Can you work these out from the model? Positions are in its coordinate system, mm. Give positions to 0.01 mm unless a question says otherwise; leave off trailing zeros. Write each loop counter-clockwise with the first axis right and the second up, starting at its lowest first coordinate (ties: lowest second). Pieces come first, ordered by that corner, then holes. Notation, with made-up numbers: (71, 45) - (122, 45) arc R6 ccw to (122, 54) - close; hole circle Ø1 at (-1, -32). An arc over 180 degrees is marked (long way). Use a Markdown table: item, result. Add a question column.
```python
from build123d import *

# Parameters (mm, degrees)
F0_R     = 25.1418135505
F1_DEPTH = 32.512
F2_T     = -2.54


# Not quite as in the source:
# - a fillet or chamfer that OpenCascade refuses, or shapes differently, is made with other operations: its cross-section is extruded or revolved along the edge and cut away or added


with BuildPart() as f1:
    # F0 (on Top) → F1 (new body)
    with BuildSketch(Plane.XY):
        Circle(F0_R)
    extrude(amount=F1_DEPTH)

    # F2
    f2_openings = [f1.faces().sort_by_distance(p)[0] for p in [
        (0, 0, 32.512),
    ]]
    offset(amount=F2_T, openings=f2_openings)

    # F3: fillet of radius 5.08 on 3 edges, made by hand

    # F3_s1 → F3_t2 (revolve, cut)
    with BuildSketch(Plane.XZ):
        with BuildLine():
            ThreePointArc((25.1418135505, 28.1125909488), (24.4612226018, 30.6525909488), (22.6018135505, 32.512))
            Line((22.6018135505, 32.512), (22.6526135505, 32.599988181))
            ThreePointArc((22.6526135505, 32.599988181), (23.8718135505, 32.6136), (25.1418135505, 32.6136))
            Line((25.1418135505, 32.6136), (25.2434135505, 32.512))
            Line((25.2434135505, 32.512), (25.2434135505, 28.1125909488))
            Line((25.2434135505, 28.1125909488), (25.1418135505, 28.1125909488))
        make_face()
    revolve(axis=Axis((0, 0, 32.512), (0, 0, 1)), mode=Mode.SUBTRACT)

    # F3_s3 → F3_t4 (revolve, cut)
    with BuildSketch(Plane.XZ):
        with BuildLine():
            ThreePointArc((25.1418135505, 5.08), (23.653915999, 1.4878975516), (20.0618135505, 0))
            Line((20.0618135505, 0), (20.0618135505, -0.1016))
            Line((20.0618135505, -0.1016), (25.2434135505, -0.1016))
            Line((25.2434135505, -0.1016), (25.2434135505, 5.08))
            Line((25.2434135505, 5.08), (25.1418135505, 5.08))
        make_face()
    revolve(axis=Axis((0, 0, 0), (0, 0, 1)), mode=Mode.SUBTRACT)


solid = f1.part
```
Q1. Suppose I cut it at A-A (x = 0). Please give me the cut outline in (y, z).
Q2. If we mould it in two halves opening along Y, with no side actions, what happens to faces 1 (the flat face through (0, 0, 0)), 2 (the flat face through (0, 0, 2.54)), 3 (the cylindrical face through (-5.45, -24.544, 16.435))? For each: released by +Y, released by -Y, zero draft, split by the parting line, or undercut.
Q3. Suppose I cut it at B-B (z = 26.5). Please give me the cut outline in (x, y), and give its area (3 significant figures).
Q4. If I drill on probe 1 along Y at (x, z) = (0, 12); probe 2 along Z at (x, y) = (8.5, -2), over which ranges is the centre line in solid material (lowest first)? Write a range as [from, to].
Q5. I'm going to push flat-ended pins straight in: P1, Ø5, axis at x = -0.5, y = 11, coming from the +Z side; P2, Ø3, axis at x = -9, z = 12, coming from the +Y side; P3, Ø5, axis at y = 1.5, z = 12, coming from the -X side; P4, Ø4, axis at y = 14, z = 6, coming from the -X side. Where does each tip first touch, or does it pass through?
Derived:
| question | item | result |
|---|---|---|
| 1 | outline | (-25.14, 5.08) arc R5.08 ccw to (-20.06, 0) - (20.06, 0) arc R5.08 ccw to (25.14, 5.08) - (25.14, 28.11) arc R5.08 ccw to (22.6, 32.51) - (22.6, 2.54) - (-22.6, 2.54) - (-22.6, 32.51) arc R5.08 ccw to (-25.14, 28.11) - close |
| 2 | face 1 | zero draft |
| 2 | face 2 | undercut |
| 2 | face 3 | split by the parting line |
| 3 | outline | circle Ø50.28 at (0, 0); hole circle Ø45.2 at (0, 0) |
| 3 | area | 381 mm² |
| 4 | probe 1 | [-25.14, -22.6], [22.6, 25.14] |
| 4 | probe 2 | [0, 2.54] |
| 5 | P1 | z = 2.54 |
| 5 | P2 | y = 24 |
| 5 | P3 | x = -25.14 |
| 5 | P4 | x = -22.09 |
